Source: CAD feature listing. Evaluate the final solid. Frame: model axes, mm. Give positions to 0.01 mm unless a question says otherwise; leave off trailing zeros. Loops run counter-clockwise (first coordinate to the right, second up) from the corner with the lowest first, then second, coordinate; pieces in that order, holes last.
from build123d import *

# Parameters (mm, degrees)
F2_R = 1


with BuildPart() as f1:
    # F0 (on Front) → F1 (revolve)
    with BuildSketch(Plane.XZ):
        with BuildLine():
            ThreePointArc((0, 50), (-1.34161, 49.609522), (-2.264125, 48.560066))
            Line((-2.264125, 48.560066), (-25, 0))
            Line((-25, 0), (0, 0))
            Line((0, 0), (0, 50))
        make_face()
    revolve(axis=Axis((0, 0, 26.697931), (0, 0, 1)))

    # F2
    f2_edges = [f1.edges().sort_by_distance(p)[0] for p in [
        (25, 0, 0),
    ]]
    fillet(f2_edges, radius=F2_R)

    # F3 (on Front) → F4 (revolve, cut)
    with BuildSketch(Plane.XZ):
        Polygon((0, 3.5), (0, 44.905821), (-19.38625, 3.5), align=None)
    revolve(axis=Axis((0, 0, 24.883967), (0, 0, -1)), mode=Mode.SUBTRACT)


solid = f1.part
1) Cut plane A-A (z = 35). Return loops of the section in (x, y), and give its area (3 significant figures).
Checks:
outline: circle Ø17.23 at (0, 0); hole circle Ø9.28 at (0, 0)
area: 165 mm2
2) Pull-direction query (Y, two-part tool) for faces 1 (the conical face through (-7.09, -2.94, 28.51)), 2 (the flat face through (0, 0, 0)), 3 (the conical face through (8.73, 6.69, 29.9)); classes: released by +Y, released by -Y, zero draft, split by the parting line, or undercut.
Checks:
face 1: undercut
face 2: zero draft
face 3: split by the parting line
3) Cut plane B-B (z = 10). Return loops of the section in (x, y).
Checks:
outline: circle Ø40.64 at (0, 0); hole circle Ø32.69 at (0, 0)
4) Ray query, probe 1 along Y at (x, z) = (8, 24.5); probe 2 along Z at (x, y) = (-19, -2); probe 3 along Z at (x, y) = (-11.5, 8). Return the intervals inside material, ascending.
Checks:
probe 1: y = -10.91 to -5.22, 5.22 to 10.91
probe 2: z = 0 to 3.5, 4.1 to 12.59
probe 3: z = 0 to 3.5, 14.99 to 23.48
5) Contact query for flat-ended pins moving along their axis: P1, Ø8, axis at x = -15.5, y = 19, coming from the -Z side; P2, Ø1, axis at x = 9, y = -5, coming from the +Z side; P3, Ø1.5, axis at x = 18.5, z = 6.5, coming from the -Y side; P4, Ø12, axis at y = 7.5, z = 38, coming from the -X side. Output: stop coordinate, or through.
Checks:
P1: stops at z = 0
P2: stops at z = 32.47
P3: stops at y = -13.08
P4: stops at x = -8.62
